Check sheet for the modelled part. Datum: model origin and axes. Units: mm. A direction names the side the tool comes from. Coordinates: 2 decimals unless noted, no trailing zeros. Write each loop counter-clockwise with the first axis right and the second up, starting at its lowest first coordinate (ties: lowest second). Pieces come first, ordered by that corner, then holes. Notation, with made-up numbers: M -26,64 L -16,64 A6 cw -16,69 Z; hole C -32.75,82 d7. An arc over 180 degrees is marked long. Answer as CSV lines item,"result". Start each with the question number.
Q1. Access from +Z, -Z, +X, -X, +Y, -Y to the whole of each face (thin tool, end or side, straight path). Record for faces 1 (the flat face through (35, 25, 3)), 2 (the flat face through (35, 76, 3)), 3 (the flat face through (0, 50, 9)).
Q2. Sectioned sample at B-B, the plane z = 37.5. Record the cut outline in (x, y).
Q3. Sectioned sample at A-A, the plane x = 19. Record the cut outline in (y, z), then the cut area to 3 significant figures.
Q4. Depth check by flat-ended pin: pin 1 Ø1 at (x, y) = (47, 90) entering from +Z; pin 2 Ø12 at (x, z) = (50, 30) entering from -Y; pin 3 Ø21 at (x, z) = (26, 27.5) entering from +Y; pin 4 Ø12 at (y, z) = (44.5, 26) entering from +X. Enter the tip coordinate at first touch or a pass-through.
Q5. Thickness scan on line 1 along Z through (x, y) = (38, 41); line 2 along Y through (x, z) = (3, 25). Record the ranges inside material, lowest first. Write a range as from..to.
Q6. Sectioned sample at C-C, the plane y = 7. Record the cut outline in (x, z).
Autodesk Fusion 360 part; units mm, degrees
sketch "Sketch1" plane through (0, 0, 0) normal (0, 0, 1) x (1, 0, 0)
  line L0 (0, 90) -> (10, 100)
  line L1 (70, 90) -> (60, 100)
  line L2 (0, 10) -> (10, 0)
  line L3 (70, 10) -> (60, 0)
  line L4 (10, 100) -> (60, 100)
  line L5 (70, 90) -> (70, 10)
  line L6 (60, 0) -> (10, 0)
  line L7 (0, 10) -> (0, 90)
  line L8 (70, 51.5) -> (0, 51.5)
  line L9 (70, 48.5) -> (0, 48.5)
extrude "Extrude1" add sketch "Sketch1" along normal blind 3 makes body 1
extrude "Extrude2" add sketch "Sketch1" along normal blind 45 separate body contours L5 L7 L8 L9 makes body 2
combine "Combine1" operation add target body 1 tool bodies 2
Output:
1,face 1,"+Z, +X, -X, -Y"
1,face 2,"+Z, +X, -X, +Y"
1,face 3,"+Z, -Z, -X, +Y, -Y"
2,outline,"M 0,48.5 L 70,48.5 L 70,51.5 L 0,51.5 Z"
3,outline,"M 0,0 L 100,0 L 100,3 L 51.5,3 L 51.5,45 L 48.5,45 L 48.5,3 L 0,3 Z"
3,area,"426 mm^2"
4,pin 1,"stops at z = 3"
4,pin 2,"stops at y = 48.5"
4,pin 3,"stops at y = 51.5"
4,pin 4,"stops at x = 70"
5,line 1,"z = 0..3"
5,line 2,"y = 48.5..51.5"
6,outline,"M 3,0 L 67,0 L 67,3 L 3,3 Z"
